Could you check a few things on this drawing? It's one solid part, dimensions in mm from its lowest x, y, z. A direction names the side the tool comes from. Give positions to 0.01 mm unless a question says otherwise; leave off trailing zeros. Write each loop counter-clockwise with the first axis right and the second up, starting at its lowest first coordinate (ties: lowest second). Pieces come first, ordered by that corner, then holes. Notation, with made-up numbers: M 14,43 L 69,43 A16 ccw 69,60 Z; hole C 54.25,2 d6. An arc over 180 degrees is marked long. Answer as CSV lines item,"result". Start each with the question number.
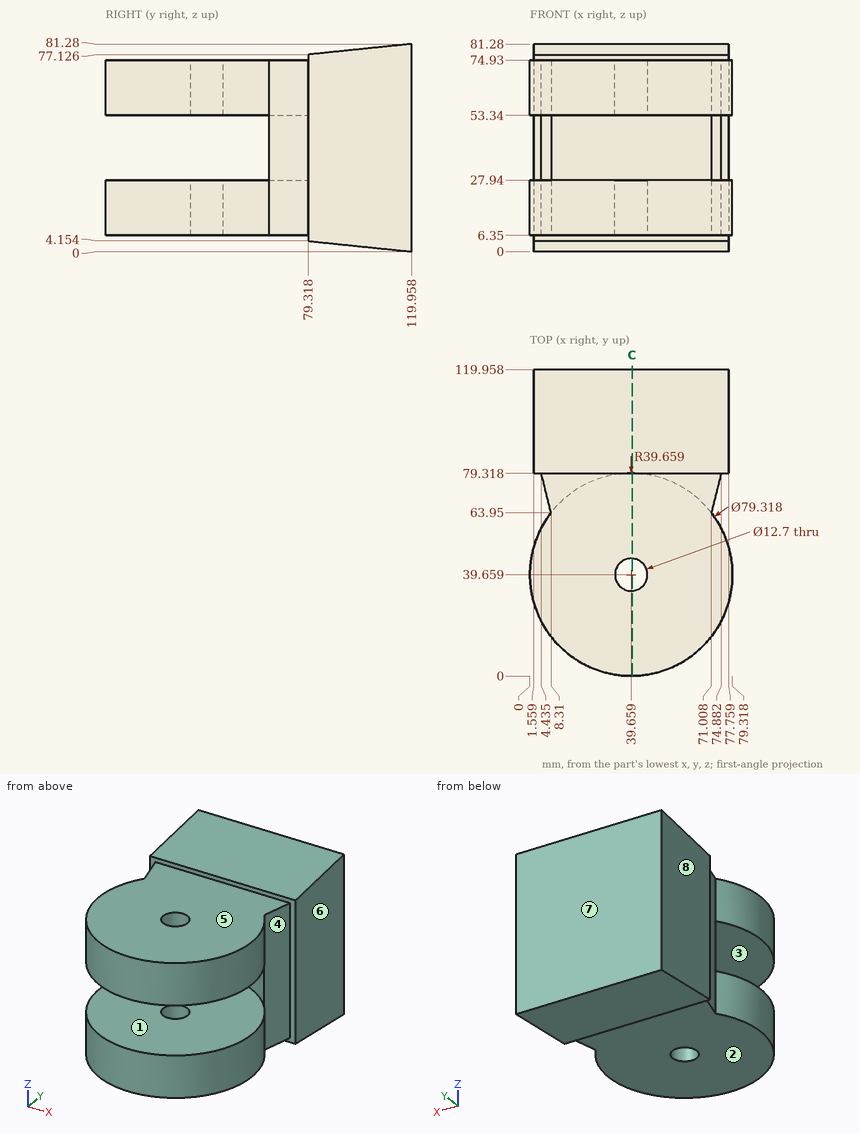
1) I need wall thicknesses on L1, parallel to Z at x = 65.5, y = 45.5; L2, parallel to X at y = 109, z = 5; L3, parallel to Z at x = 72, y = 72. Which ranges of each line are inside material? Lowest first, please. Write a range as from..to.
2) On a 3-axis mill with a long thin cutter (end or side, diameter ignored), from which of +Z, -Z, +X, -X, +Y, -Y can I reach the whole of each face in a straight line? I mean the marked faces 5, 6, 7 and 8. Say none if no direction works.
3) I'm going to push flat-ended pins straight in: P1, Ø1.5, axis at y = 100, z = 69, coming from the -X side; P2, Ø8, axis at y = 33.5, z = 64.5, coming from the +X side; P3, Ø16.5, axis at x = 39.66, y = 39.66, coming from the +Z side. Where does each tip first touch, or does it pass through?
4) I want a section at C-C, the plane x = 40. Please give me the cut outline in (y, z).
5) Thinking about a two-plate mould opening in X: for the marked faces 1, 2, 3 and 4, which applies, released by +X, released by -X, zero draft, split by the parting line, or undercut?
Values found:
1,L1,"z = 6.35..27.94, 53.34..74.93"
1,L2,"x = 1.56..77.76"
1,L3,"z = 6.35..74.93"
2,face 5,"+Z, +X, -X, -Y"
2,face 6,"+Z, -Z, +X, +Y"
2,face 7,"+Z, -Z, +X, -X, +Y"
2,face 8,"+Z, -Z, -X, +Y"
3,P1,"stops at x = 1.56"
3,P2,"stops at x = 79.26"
3,P3,"stops at z = 74.93"
4,outline,"M 0,6.35 L 33.32,6.35 L 33.32,27.94 L 0,27.94 Z; M 0,53.34 L 33.32,53.34 L 33.32,74.93 L 0,74.93 Z; M 46,6.35 L 79.32,6.35 L 79.32,4.15 L 119.96,0 L 119.96,81.28 L 79.32,77.13 L 79.32,74.93 L 46,74.93 L 46,53.34 L 79.32,53.34 L 79.32,27.94 L 46,27.94 Z"
5,face 1,"undercut"
5,face 2,"zero draft"
5,face 3,"undercut"
5,face 4,"released by +X"
